Read the model definition and answer for the solid it produces. Units are mm, in the model's axes. Face numbers are marked on the shaded views. Coordinates: 2 decimals unless noted, no trailing zeros. Write each loop counter-clockwise with the first axis right and the second up, starting at its lowest first coordinate (ties: lowest second). Pieces come first, ordered by that corner, then holes. Notation, with made-up numbers: (5, -35) -> (32, -35) arc R22 ccw to (32, 1) -> close; hole circle Ø7 at (11.25, 55). An arc over 180 degrees is marked (long way). Answer in a Markdown table with one row per item. Add a question column.
Item 1: Section A-A on z = 5 is taken. Write down the section's boundary in (x, y), then the cut area to 3 significant figures.
Item 2: For a pull along Z with two mould halves and no side action, classify the marked faces 1, 2 and 3 as +Z half, -Z half, draft (parallel to the pull), parting line (faces both ways), or undercut.
Item 3: Section C-C on y = 1.75 is taken. Write down the section's boundary in (x, z), then the cut area to 3 significant figures.
Item 4: Straight lines are drawn through the part: line 1 (Y direction, x = 1.75, z = 8); line 2 (Z direction, x = 4.5, y = 8); line 3 (Z direction, x = 3, y = 16.25). For each, find the intervals that lie inside material, in ascending order. Write a range as from..to.
Item 5: Section D-D on x = -4.25 is taken. Write down the section's boundary in (y, z).
Item 6: Given pin 1 Ø0.5 at (x, z) = (-0.5, -14) entering from +Y; pin 2 Ø3 at (y, z) = (13, 26) entering from -X; pin 3 Ø6.5 at (x, z) = (-0.5, -4) entering from +Y, each flat-ended and moving along its own axis, determine where each tip first touches the part or whether it passes through.
Item 7: Section B-B on x = 0 is taken. Count the separate pieces of the cut face and the enclosed holes in it, then the cut area to 3 significant figures.
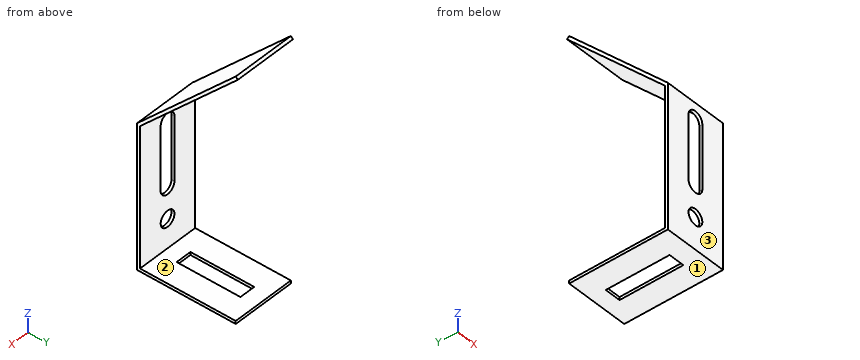
```python
from build123d import *

# Parameters (mm, degrees)
SKETCH1_W           = 12.7
SKETCH1_H           = 28.575
SKETCH1_R           = 1.5875
BOSS_EXTRUDE1_DEPTH = 0.5953125
SKETCH3_W           = 12.7
SKETCH3_H           = 19.05
SKETCH3_W_2         = 3.175
SKETCH3_H_2         = 12.7
BOSS_EXTRUDE2_DEPTH = 0.5953125
BOSS_EXTRUDE3_DEPTH = 12.7


with BuildPart() as part:
    # Sketch1 → Boss-Extrude1 (new body)
    with BuildSketch(Plane(origin=(0, 0, 0), x_dir=(1, 0, 0), z_dir=(0, 1, 0))):
        Rectangle(SKETCH1_W, SKETCH1_H)
        with Locations(Location((0, 7.9375, 0), (0, 0, 90))):
            Circle(SKETCH1_R, mode=Mode.SUBTRACT)
        with BuildLine():
            Line((1.5875, 1.5875), (1.5875, -11.1125))
            ThreePointArc((1.5875, -11.1125), (0, -12.7), (-1.5875, -11.1125))
            Line((-1.5875, -11.1125), (-1.5875, 1.5875))
            ThreePointArc((-1.5875, 1.5875), (0, 3.175), (1.5875, 1.5875))
        make_face(mode=Mode.SUBTRACT)
    extrude(amount=BOSS_EXTRUDE1_DEPTH)

    # Sketch3 → Boss-Extrude2 (add)
    with BuildSketch(Plane(origin=(0, 0, -14.2875), x_dir=(-1, 0, 0), z_dir=(0, 0, -1))):
        with Locations((0, 10.1203125)):
            Rectangle(SKETCH3_W, SKETCH3_H)
        with Locations((0, 10.1203125)):
            Rectangle(SKETCH3_W_2, SKETCH3_H_2, mode=Mode.SUBTRACT)
    extrude(amount=-BOSS_EXTRUDE2_DEPTH)

    # Sketch4 → Boss-Extrude3 (add)
    with BuildSketch(Plane(origin=(6.35, 0, 0), x_dir=(0, 0, -1), z_dir=(1, 0, 0))):
        Polygon((-14.2875, 0), (-33.9328125, 19.6453125), (-33.511862994, 20.066262006), (-14.040913489, 0.5953125), (-14.2875, 0.5953125), align=None)
    extrude(amount=-BOSS_EXTRUDE3_DEPTH)


solid = part.part
```
Results below:
| question | item | result |
|---|---|---|
| 1 | outline | (-6.35, 0) -> (-1.59, 0) -> (-1.59, 0.6) -> (-6.35, 0.6) -> close; (1.59, 0) -> (6.35, 0) -> (6.35, 0.6) -> (1.59, 0.6) -> close |
| 1 | area | 5.67 mm2 |
| 2 | face 1 | -Z half |
| 2 | face 2 | undercut |
| 2 | face 3 | draft |
| 3 | outline | (-6.35, -14.29) -> (6.35, -14.29) -> (6.35, -13.69) -> (-6.35, -13.69) -> close; (-6.35, 15.2) -> (6.35, 15.2) -> (6.35, 16.04) -> (-6.35, 16.04) -> close |
| 3 | area | 18.3 mm2 |
| 4 | line 1 | y = 0..0.6 |
| 4 | line 2 | z = -14.29..-13.69, 21.45..22.29 |
| 4 | line 3 | z = -14.29..-13.69, 29.7..30.54 |
| 5 | outline | (0, -14.29) -> (19.65, -14.29) -> (19.65, -13.69) -> (0.6, -13.69) -> (0.6, 14.04) -> (20.07, 33.51) -> (19.65, 33.93) -> (0, 14.29) -> close |
| 6 | pin 1 | stops at y = 19.65 |
| 6 | pin 2 | stops at x = -6.35 |
| 6 | pin 3 | stops at y = 0.6 |
| 7 | separate pieces | 4 |
| 7 | enclosed holes | 0 |
| 7 | area | 25.8 mm2 |
